CAD build for the part. Positions are in the model's coordinates, mm. A direction names the side the tool comes from. Round coordinates to 2 decimals unless told otherwise and drop trailing zeros. Order: outer loops, then holes, each group sorted by start corner. A loop starts at its lowest first (then second) coordinate and runs counter-clockwise, first axis right, second up.
```python
from build123d import *

# Parameters (mm, degrees)
EXTRUDE_4_DEPTH = 70
EXTRUDE_START   = -5
EXTRUDE_5_DEPTH = 5


with BuildPart() as part:
    # 草图1 → 凸台-拉伸4 (new body)
    with BuildSketch(Plane.XY):
        with BuildLine():
            Line((-52.598076211, -29), (-50, -30.5))
            Line((-50, -30.5), (-50, 35.5))
            Line((-50, 35.5), (-38.637956343, 73.373478856))
            ThreePointArc((-38.637956343, 73.373478856), (-35.028998787, 78.522929283), (-29.059693491, 80.5))
            Line((-29.059693491, 80.5), (0, 80.5))
            Line((0, 80.5), (29.059693491, 80.5))
            ThreePointArc((29.059693491, 80.5), (35.028998787, 78.522929283), (38.637956343, 73.373478856))
            Line((38.637956343, 73.373478856), (50, 35.5))
            Line((50, 35.5), (50, -30.5))
            Line((50, -30.5), (52.598076211, -29))
            Line((52.598076211, -29), (52.598076211, -34))
            Line((52.598076211, -34), (50, -32.5))
            Line((50, -32.5), (50, -35.5))
            Line((50, -35.5), (55, -35.5))
            Line((55, -35.5), (55, 34.032311637))
            ThreePointArc((55, 34.032311637), (54.894003955, 35.484443084), (54.578262852, 36.905790493))
            Line((54.578262852, 36.905790493), (42.137956343, 78.373478856))
            ThreePointArc((42.137956343, 78.373478856), (38.528998787, 83.522929283), (32.559693491, 85.5))
            Line((32.559693491, 85.5), (0, 85.5))
            Line((0, 85.5), (-32.559693491, 85.5))
            ThreePointArc((-32.559693491, 85.5), (-38.528998787, 83.522929283), (-42.137956343, 78.373478856))
            Line((-42.137956343, 78.373478856), (-54.578262852, 36.905790493))
            ThreePointArc((-54.578262852, 36.905790493), (-54.894003955, 35.484443084), (-55, 34.032311637))
            Line((-55, 34.032311637), (-55, -35.5))
            Line((-55, -35.5), (-50, -35.5))
            Line((-50, -35.5), (-50, -32.5))
            Line((-50, -32.5), (-52.598076211, -34))
            Line((-52.598076211, -34), (-52.598076211, -29))
        make_face()
    extrude(amount=EXTRUDE_4_DEPTH)

    # 草图2 → 凸台-拉伸5 (add)
    with BuildSketch(Plane.XY.offset(70).offset(EXTRUDE_START)):
        with BuildLine():
            Line((-50, -35.5), (50, -35.5))
            Line((50, -35.5), (50, -32.5))
            Line((50, -32.5), (52.598076211, -34))
            Line((52.598076211, -34), (52.598076211, -29))
            Line((52.598076211, -29), (50, -30.5))
            Line((50, -30.5), (50, 35.5))
            Line((50, 35.5), (38.637956343, 73.373478856))
            ThreePointArc((38.637956343, 73.373478856), (35.028998787, 78.522929283), (29.059693491, 80.5))
            Line((29.059693491, 80.5), (-29.059693491, 80.5))
            ThreePointArc((-29.059693491, 80.5), (-35.028998787, 78.522929283), (-38.637956343, 73.373478856))
            Line((-38.637956343, 73.373478856), (-50, 35.5))
            Line((-50, 35.5), (-50, -30.5))
            Line((-50, -30.5), (-52.598076211, -29))
            Line((-52.598076211, -29), (-52.598076211, -34))
            Line((-52.598076211, -34), (-50, -32.5))
            Line((-50, -32.5), (-50, -35.5))
        make_face()
    extrude(amount=EXTRUDE_5_DEPTH)


solid = part.part
```
1. Cut at A-A, the plane z = 20.5. Write the cut outline in (x, y), and give its area (3 significant figures).
2. Cut at D-D, the plane y = 48. Write the cut outline in (x, z), and give its area (3 significant figures).
3. Drill centre lines: line 1 (X direction, y = 5, z = 11); line 2 (Y direction, x = 24.5, z = 11); line 3 (Z direction, x = -11.5, y = -10). Where is each one in solid material? Low to high.
4. Mould opens along X. For faces 3 (the face through (0, 84, 0)), 4 (the face through (-35.1, 78.47, 32.04)), 5 (the face through (-55, 0, 35)) say: released by +X, released by -X, zero draft, split by the parting line, or undercut.
5. Cut at B-B, the plane y = 16.5. Write the cut outline in (x, z).
6. Cut at C-C, the plane x = -7. Write the cut outline in (y, z), and give its area (3 significant figures).
7. Tool access for faces 1 (the face through (44.24, 54.7, 32.04)), 2 (the face through (38.6, 83.47, 34.51)): list every direction of +Z, -Z, +X, -X, +Y, -Y with a clear straight run to the whole face (end or side of a thin tool).
8. Pin check, flat tips, straight feed: P1, Ø3, axis at x = 18.5, z = 46.5, coming from the -Y side; P2, Ø2, axis at x = -34, z = 29.5, coming from the +Y side; P3, Ø6, axis at x = 40, y = -4, coming from the -Z side. Stop position of each tip, or through.
Outcome:
1. outline: (-55, -35.5) - (-50, -35.5) - (-50, -32.5) - (-52.6, -34) - (-52.6, -29) - (-50, -30.5) - (-50, 35.5) - (-38.64, 73.37) arc R10 cw to (-29.06, 80.5) - (29.06, 80.5) arc R10 cw to (38.64, 73.37) - (50, 35.5) - (50, -30.5) - (52.6, -29) - (52.6, -34) - (50, -32.5) - (50, -35.5) - (55, -35.5) - (55, 34.03) arc R10 ccw to (54.58, 36.91) - (42.14, 78.37) arc R10 ccw to (32.56, 85.5) - (-32.56, 85.5) arc R10 ccw to (-42.14, 78.37) - (-54.58, 36.91) arc R10 ccw to (-55, 34.03) - close
1. area: 1,550 mm2
2. outline: (-51.25, 0) - (-46.25, 0) - (-46.25, 65) - (46.25, 65) - (46.25, 0) - (51.25, 0) - (51.25, 70) - (-51.25, 70) - close
2. area: 1,160 mm2
3. line 1: x = -55 to -50, 50 to 55
3. line 2: y = 80.5 to 85.5
3. line 3: z = 65 to 70
4. face 3: zero draft
4. face 4: undercut
4. face 5: released by -X
5. outline: (-55, 0) - (-50, 0) - (-50, 65) - (50, 65) - (50, 0) - (55, 0) - (55, 70) - (-55, 70) - close
6. outline: (-35.5, 65) - (80.5, 65) - (80.5, 0) - (85.5, 0) - (85.5, 70) - (-35.5, 70) - close
6. area: 930 mm2
7. face 1: -Z, -Y
7. face 2: +Z, -Z, +X, +Y
8. P1: stops at y = 80.5
8. P2: stops at y = 85.49
8. P3: stops at z = 65
